Input: part model. Units: mm. Frame: model coordinates. Face numbers are marked on the shaded views. A direction names the side the tool comes from. Coordinates: 2 decimals unless noted, no trailing zeros. Order: outer loops, then holes, each group sorted by start corner. A loop starts at its lowest first (then second) coordinate and runs counter-clockwise, first axis right, second up. Notation, with made-up numbers: (32, 60.5) - (83, 60.5) arc R30 ccw to (83, 87.5) - close; hole circle Ø4 at (-32, 20.5). An arc over 180 degrees is marked (long way). One line per question, with ' | ' between items.
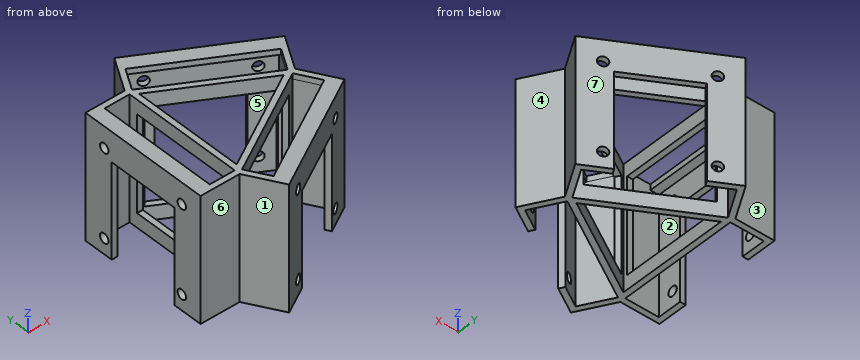
from build123d import *

# Parameters (mm, degrees)
PAD_DEPTH       = 44
PAD001_DEPTH    = 11.8
SKETCH002_R     = 1.7
PAD002_DEPTH    = 2
POCKET_DEPTH    = 5
SKETCH004_W     = 36
SKETCH004_H     = 34
POCKET001_DEPTH = 3
SKETCH005_W     = 36
SKETCH005_H     = 34
POCKET002_DEPTH = 4
PAD003_DEPTH    = 11.8
SKETCH007_R     = 1.7
PAD004_DEPTH    = 2
POCKET003_DEPTH = 2
PAD005_DEPTH    = 11.8
SKETCH010_R     = 1.7
PAD006_DEPTH    = 2
SKETCH011_W     = 8.8
SKETCH011_H     = 42
POCKET004_DEPTH = 2
SKETCH012_W     = 36
SKETCH012_H     = 34
POCKET005_DEPTH = 3


with BuildPart() as part:
    # Sketch → Pad (new body)
    with BuildSketch(Plane.XY):
        Polygon((26.5581123827, 0), (-13.2790561914, 23), (-13.2790561914, -23), align=None)
        Polygon((22.5166604984, 0), (-11.2583302492, 19.5), (-11.2583302492, -19.5), align=None, mode=Mode.SUBTRACT)
    extrude(amount=PAD_DEPTH)

    # Sketch001 (on Face3 of Pad) → Pad001 (join)
    with BuildSketch(Plane(origin=(6.6395280957, -11.5, 0), x_dir=(0.8660254038, 0.5, 0), z_dir=(0.5, -0.8660254038, 0))):
        Polygon((-23, 0), (-21, 0), (-21, 42), (21, 42), (21, 0), (23, 0), (23, 44), (-23, 44), align=None)
    extrude(amount=PAD001_DEPTH)

    # Sketch002 (on Face8 of Pad001) → Pad002 (join)
    with BuildSketch(Plane(origin=(12.5395280957, -21.7190997647, 0), x_dir=(0.8660254038, 0.5, 0), z_dir=(0.5, -0.8660254038, 0))):
        Polygon((-23, 0), (-12.5, 0), (-12.5, 33.5), (12.5, 33.5), (12.5, 0), (23, 0), (23, 44), (-23, 44), align=None)
        with Locations((-15.5, 36.5)):
            Circle(SKETCH002_R, mode=Mode.SUBTRACT)
        with Locations((-15.5, 5.5)):
            Circle(SKETCH002_R, mode=Mode.SUBTRACT)
        with Locations((15.5, 5.5)):
            Circle(SKETCH002_R, mode=Mode.SUBTRACT)
        with Locations((15.5, 36.5)):
            Circle(SKETCH002_R, mode=Mode.SUBTRACT)
    extrude(amount=PAD002_DEPTH)

    # Sketch003 (on Face7 of Pad002) → Pocket (cut)
    with BuildSketch(Plane.XY.offset(44)):
        Polygon((-11.5470053838, -22), (-7.1470053838, -29.6210235533), (29.2260615752, -8.6210235533), (24.8260615752, -1), align=None)
    extrude(amount=-POCKET_DEPTH, mode=Mode.SUBTRACT)

    # Sketch004 (on Face11 of Pocket) → Pocket001 (cut)
    with BuildSketch(Plane(origin=(6.6395280957, -11.5, 0), x_dir=(0.8660254038, 0.5, 0), z_dir=(0.5, -0.8660254038, 0))):
        with Locations((0, 22)):
            Rectangle(SKETCH004_W, SKETCH004_H)
    extrude(amount=-POCKET001_DEPTH, mode=Mode.SUBTRACT)

    # Sketch005 (on Face1 of Pocket001) → Pocket002 (cut)
    with BuildSketch(Plane(origin=(6.6395280957, 11.5, 0), x_dir=(-0.8660254038, 0.5, 0), z_dir=(0.5, 0.8660254038, 0))):
        with Locations((0, 22)):
            Rectangle(SKETCH005_W, SKETCH005_H)
    extrude(amount=-POCKET002_DEPTH, mode=Mode.SUBTRACT)

    # Sketch006 (on Face1 of Pocket002) → Pad003 (join)
    with BuildSketch(Plane(origin=(6.6395280957, 11.5, 0), x_dir=(-0.8660254038, 0.5, 0), z_dir=(0.5, 0.8660254038, 0))):
        Polygon((-23, 44), (23, 44), (23, 0), (21, 0), (21, 42), (-21, 42), (-21, 0), (-23, 0), align=None)
    extrude(amount=PAD003_DEPTH)

    # Sketch007 (on Face19 of Pad003) → Pad004 (join)
    with BuildSketch(Plane(origin=(12.5395280957, 21.7190997647, 0), x_dir=(-0.8660254038, 0.5, 0), z_dir=(0.5, 0.8660254038, 0))):
        Polygon((-23, 0), (-12.5, 0), (-12.5, 33.5), (12.5, 33.5), (12.5, 0), (23, 0), (23, 44), (-23, 44), align=None)
        with Locations((-15.5, 36.5)):
            Circle(SKETCH007_R, mode=Mode.SUBTRACT)
        with Locations((15.5, 36.5)):
            Circle(SKETCH007_R, mode=Mode.SUBTRACT)
        with Locations((15.5, 5.5)):
            Circle(SKETCH007_R, mode=Mode.SUBTRACT)
        with Locations((-15.5, 5.5)):
            Circle(SKETCH007_R, mode=Mode.SUBTRACT)
    extrude(amount=PAD004_DEPTH)

    # Sketch008 (on Face43 of Pad004) → Pocket003 (cut)
    with BuildSketch(Plane.XY.offset(44)):
        Polygon((-11.5470053838, 22), (-7.1470053838, 29.6210235533), (29.2260615751, 8.6210235533), (24.8260615752, 1), align=None)
    extrude(amount=-POCKET003_DEPTH, mode=Mode.SUBTRACT)

    # Sketch009 (on Face12 of Pocket003) → Pad005 (join)
    with BuildSketch(Plane(origin=(-13.2790561914, 0, 0), x_dir=(0, -1, 0), z_dir=(-1, 0, 0))):
        Polygon((-23, 0), (-21, 0), (-21, 42), (21, 42), (21, 0), (23, 0), (23, 44), (-23, 44), align=None)
    extrude(amount=PAD005_DEPTH)

    # Sketch010 (on Face32 of Pad005) → Pad006 (join)
    with BuildSketch(Plane(origin=(-25.0790561914, 0, 0), x_dir=(0, -1, 0), z_dir=(-1, 0, 0))):
        Polygon((-23, 0), (-12.5, 0), (-12.5, 33.5), (12.5, 33.5), (12.5, 0), (23, 0), (23, 44), (-23, 44), align=None)
        with Locations((-15.5, 5.5)):
            Circle(SKETCH010_R, mode=Mode.SUBTRACT)
        with Locations((-15.5, 36.5)):
            Circle(SKETCH010_R, mode=Mode.SUBTRACT)
        with Locations((15.5, 36.5)):
            Circle(SKETCH010_R, mode=Mode.SUBTRACT)
        with Locations((15.5, 5.5)):
            Circle(SKETCH010_R, mode=Mode.SUBTRACT)
    extrude(amount=PAD006_DEPTH)

    # Sketch011 (on Face57 of Pad006) → Pocket004 (cut)
    with BuildSketch(Plane.XY.offset(44)):
        with Locations((-17.6790561914, 0)):
            Rectangle(SKETCH011_W, SKETCH011_H)
    extrude(amount=-POCKET004_DEPTH, mode=Mode.SUBTRACT)

    # Sketch012 (on Face13 of Pocket004) → Pocket005 (cut)
    with BuildSketch(Plane(origin=(-13.2790561914, 0, 0), x_dir=(0, -1, 0), z_dir=(-1, 0, 0))):
        with Locations((0, 22)):
            Rectangle(SKETCH012_W, SKETCH012_H)
    extrude(amount=-POCKET005_DEPTH, mode=Mode.SUBTRACT)


solid = part.part
Item 1: Access query for the marked faces 4, 5, 6 and 7. Directions: +Z, -Z, +X, -X, +Y, -Y. A direction counts if a zero-diameter tool reaches every point of the face in a straight line with its end or side. Return the directions, or none.
Data:
face 4: +Z, -Z, +X | face 5: -Z | face 6: +Z, -Z, -X, -Y | face 7: +Z, -Z, +X, +Y
Item 2: Section D-D on x = 9. Return the cut outline in (y, z).
Data:
outline: (-26.07, 33.5) - (-23.76, 33.5) - (-23.76, 42) - (-20.3, 42) - (-20.3, 44) - (-26.07, 44) - close; (-10.14, 0) - (-7.8, 0) - (-7.8, 5) - (-10.14, 5) - close; (-10.14, 39) - (-7.8, 39) - (-7.8, 44) - (-10.14, 44) - close; (7.8, 0) - (10.14, 0) - (10.14, 5) - (7.8, 5) - close; (7.8, 39) - (10.14, 39) - (10.14, 44) - (7.8, 44) - close; (20.3, 42) - (23.76, 42) - (23.76, 33.5) - (26.07, 33.5) - (26.07, 44) - (20.3, 44) - close
Item 3: Ray query, line 1 (Z direction, x = -26.35, y = 15.5); line 2 (Y direction, x = -10.5, z = 20); line 3 (Y direction, x = -19.5, z = 14). Return the intervals inside material, ascending.
Data:
line 1: 0 to 3.8, 7.2 to 34.8, 38.2 to 44 | line 2: -27.81 to -23.81, -21.4 to -19.06, 19.06 to 21.4, 23.81 to 27.81 | line 3: -23 to -21, 21 to 23
Item 4: Contact query for flat-ended pins moving along their axis: P1, Ø9.5, axis at x = -19, z = 30.5, coming from the -Y side; P2, Ø8, axis at y = 7.5, z = 12.5, coming from the -X side; P3, Ø8, axis at x = 24, z = 27.5, coming from the -Y side; P4, Ø1, axis at x = 25.5, y = 7, coming from the -Z side. Output: stop coordinate, or through.
Data:
P1: y = -23 | P2: x = 26.27 | P3: y = -17.2 | P4: through
Item 5: Section A-A on x = -20. Return the cut outline in (y, z), and give its area (3 significant figures).
Data:
outline: (-23, 0) - (-21, 0) - (-21, 44) - (-23, 44) - close; (21, 0) - (23, 0) - (23, 44) - (21, 44) - close | area: 176 mm^2
Item 6: Section C-C on y = -6.5. Return the cut outline in (x, z).
Data:
outline: (-27.08, 33.5) - (-25.08, 33.5) - (-25.08, 42) - (-22.08, 42) - (-22.08, 44) - (-27.08, 44) - close; (-13.28, 0) - (-11.26, 0) - (-11.26, 5) - (-13.28, 5) - close; (-13.28, 39) - (-11.26, 39) - (-11.26, 44) - (-13.28, 44) - close; (11.26, 0) - (15.3, 0) - (15.3, 5) - (11.26, 5) - close; (11.26, 39) - (15.3, 39) - (15.3, 44) - (11.26, 44) - close; (28, 0) - (30.31, 0) - (30.31, 44) - (28, 44) - close
Item 7: Section B-B on z = 40. Return the cut outline in (x, y), and give its area (3 significant figures).
Data:
outline: (-27.08, -23) - (-13.28, -23) - (-6.38, -34.95) - (33.46, -11.95) - (26.56, 0) - (33.46, 11.95) - (-6.38, 34.95) - (-13.28, 23) - (-27.08, 23) - close; hole (-25.08, -21) - (-13.28, -21) - (-13.28, 21) - (-25.08, 21) - close; hole (-11.55, -22) - (-5.65, -32.22) - (30.73, -11.22) - (24.83, -1) - close; hole (-11.55, 22) - (24.83, 1) - (30.73, 11.22) - (-5.65, 32.22) - close; hole (-11.26, -19.5) - (22.52, 0) - (-11.26, 19.5) - close | area: 675 mm^2
Item 8: Draft query along X for the marked faces 1, 2 and 3. Return one class per face: released by +X, released by -X, zero draft, split by the parting line, or undercut.
Data:
face 1: released by -X | face 2: undercut | face 3: zero draft
